Verification items for the finished model (mm, model axes). A direction names the side the tool comes from. Round coordinates to 2 decimals unless told otherwise and drop trailing zeros. Write each loop counter-clockwise with the first axis right and the second up, starting at its lowest first coordinate (ties: lowest second). Pieces come first, ordered by that corner, then holes. Notation, with made-up numbers: M 9.25,-35 L 25.25,-35 A32 cw 25.25,-5 Z; hole C 64.25,24 d5. An arc over 180 degrees is marked long. One line per item, written item: value. Start each with the question number.
Item 1: Gauge pin test, flat ends, axial feed: pin 1 (1 mm diameter, centred on x = 6.5, y = 1.5, fed in from +Z); pin 2 (1.5 mm diameter, centred on x = 8, y = -0.5, fed in from +Z); pin 3 (1 mm diameter, centred on x = 12.5, z = -1, fed in from -Y). Record the tip position at first contact, or that the pin passes through.
Item 2: Section check A-A, the plane x = 3.5. Record the cut outline in (y, z), then the cut area to 3 significant figures.
Item 3: Thickness scan on probe 1 along X at (y, z) = (-2.35, 0.6); probe 2 along Z at (x, y) = (15.75, -0.05); probe 3 along Z at (x, y) = (4.75, -0.4). Record the ranges inside material, lowest first. Write a range as from..to.
Item 4: Draft check along Z on faces 1 (the face through (-1.369, -0.596, 2.685)), 2 (the face through (-2.3, 0.63, 1.08)), 3 (the face through (-3, -1.1, 1.1)). Enter one of: +Z half, -Z half, draft (parallel to the pull), parting line (faces both ways), or undercut.
Item 5: Tool access check on faces 4 (the face through (8.77, -1.5, -0.07)), 5 (the face through (18, 0, 0)), 6 (the face through (-2, -1.25, 0)). Record the directions out of +Z, -Z, +X, -X, +Y, -Y that give a thin tool (end or side, any length) a straight path to the whole face; none if there is none.
Autodesk Inventor part; units mm, degrees
ref_plane "Work Plane1" through (29, 0, 0) normal (0, -1, 0) x (1, 0, 0)
ref_plane "YZ Plane" through (0, 0, 0) normal (1, 0, 0) x (0, 1, 0)
ref_plane "XZ Plane" through (0, 0, 0) normal (0, 1, 0) x (-1, 0, 0)
sketch "Sketch1" plane through (0, 0, 0) normal (0, 0, 1) x (1, 0, 0)
  line L0 (-0.8667, 0) -> (18, 0)
  line L1 (18, 0) -> (18, 1.5)
  line L2 (18, 1.5) -> (11.25, 1.5)
  line L3 (11.25, 1.5) -> (10.9432, 1.5)
  line L4 (10.9432, 1.5) -> (0, 1.5)
  line L5 (0, 1.5) -> (0, 2.75)
  line L6 (0, 2.75) -> (-3, 2.75)
  line L7 (-3, 2.75) -> (-3, 1.4434)
  line L8 (-3, 1.4434) -> (-1.7, 1.4434)
  line L9 (-1.7, 1.4434) -> (-0.8667, 0)
  line L10 (-7.2, 0) -> (22.2, 0)
  line L11 (0, -0.55) -> (0, 3.3)
  line L12 (11.25, 1.5) -> (0, 1.5) construction
  dimension "d1" = 6.75
  dimension "d2" = 0.3068
  dimension "d3" = 3
  dimension "d4" = 1.3
  dimension "d5" = 60
  dimension "d6" = 3
  dimension "d7" = 3
  dimension "d8" = 2.8868
  dimension "d9" = 5.5
  dimension "d26" = 18
revolve "Body" add sketch "Sketch1" angle 360 about axis through (-0.8667, 0, 0) along (1, 0, 0)
sketch "Sketch2" plane through (-3, 0, 0) normal (-1, 0, 0) x (0, 0, 1)
  circle A0 centre (0, 0) radius 1.4434
  line L0 (0, -3.85) -> (0, 3.85)
  line L1 (-3.85, 0) -> (3.85, 0)
  line L2 (1.4434, 0) -> (0.7217, -1.25)
  line L3 (0.7217, -1.25) -> (-0.7217, -1.25)
  line L4 (-0.7217, -1.25) -> (-1.4434, 0)
  line L5 (-1.4434, 0) -> (-0.7217, 1.25)
  line L6 (-0.7217, 1.25) -> (0.7217, 1.25)
  line L7 (0.7217, 1.25) -> (1.4434, 0)
extrude "Slot" add sketch "Sketch2" against normal up to next contours L7 A0 | A0 L2 | L6 L0 A0 | A0 L0 L3 | L0 L6 A0 | A0 L3 L0 | L4 A0 | A0 L5
fillet "Fillet1" radius 0.3 1 edges at (-3, -2.75, 0)
thread "Thread"
chamfer "Chamfer1" distance 0.3067 distance2 0.3067 1 edges at (18, -1.5, 0) measured on face at (18, -0.4645, -0.4115)
ref_plane "Work Plane1" through (29, 0, 0) normal (0, -1, 0) x (1, 0, 0)
fillet "Fillet2" radius 0.1 1 edges at (0, -1.5, 0)
equation "\"d1\" = GEL"
equation "\"d3\" = KOH"
equation "\"d4\" = INTI"
equation "\"d6\" = GD"
equation "\"d7\" = BDM"
equation "\"d8\" = 1.1547 * SW"
equation "\"d9\" = KOD"
equation "\"d30\" = R"
equation "\"d17\" = RR"
equation "\"d13\" = GEL"
equation "\"d15\" = -0.5 * SPD + 0.5 * GD"
equation "\"d16\" = GUL"
equation "\"GD\" = NND"
equation "\"NLG\" = 8"
equation "\"GEL\" = 6.75"
equation "\"KOD\" = 5.5"
equation "\"KOH\" = NND"
equation "\"INTI\" = 1.3"
equation "\"GAL\" = 0.61345 * PTC"
equation "\"GUL\" = 0.61345 * PTC"
equation "\"BDM\" = NND"
equation "\"SW\" = 2.5"
equation "\"RR\" = 0.1 * NND"
equation "\"SPD\" = NND - 1.2269 * PTC"
equation "\"R\" = 0.1"
equation "\"PHH\" = 0.13"
equation "\"GD1\" = THREADDIA - 1.2269 * PTC"
equation "\"THREADDIA\" = 3"
equation "\"FAWI\" = 45deg"
equation "\"PTC\" = 0.5"
equation "\"KOH1\" = 2.7"
equation "\"NND\" = 3"
equation "\"TOA\" = 30deg"
equation "\"E0\" = 1.155 * SW"
properties part number "AS 1420 - 1973 - M3 x 8" material "Steel, Mild"
Response values:
1. pin 1: stops at z = 1.12
1. pin 2: stops at z = 1.5
1. pin 3: stops at y = -1.41
2. outline: C 0,0 d3
2. area: 7.07 mm2
3. probe 1: x = -3..0
3. probe 2: z = -1.5..1.5
3. probe 3: z = -1.45..1.45
4. face 1: parting line
4. face 2: undercut
4. face 3: draft
5. face 4: +X
5. face 5: +Z, -Z, +X, +Y, -Y
5. face 6: -X
